from build123d import *

# Parameters (mm, degrees)
SKETCH1_W           = 863.6
SKETCH1_H           = 88.9
BOSS_EXTRUDE1_DEPTH = 38.1
SKETCH3_W           = 88.9
SKETCH3_H           = 38.1
CUT_EXTRUDE1_DEPTH  = 39.1
SKETCH4_W           = 180.975
SKETCH4_H           = 19.05
CUT_EXTRUDE2_DEPTH  = 39.1


with BuildPart() as part:
    # Sketch1 → Boss-Extrude1 (new body)
    with BuildSketch(Plane(origin=(0, 0, 0), x_dir=(1, 0, 0), z_dir=(0, 1, 0))):
        with Locations((431.8, 44.45)):
            Rectangle(SKETCH1_W, SKETCH1_H)
    extrude(amount=BOSS_EXTRUDE1_DEPTH)

    # Sketch3 → Cut-Extrude1 (cut, through all)
    with BuildSketch(Plane(origin=(0, 38.1, 0), x_dir=(1, 0, 0), z_dir=(0, 1, 0))):
        with Locations((44.45, 69.85)):
            Rectangle(SKETCH3_W, SKETCH3_H)
        with Locations((819.15, 69.85)):
            Rectangle(SKETCH3_W, SKETCH3_H)
    extrude(amount=-CUT_EXTRUDE1_DEPTH, mode=Mode.SUBTRACT)

    # Sketch4 → Cut-Extrude2 (cut, through all)
    with BuildSketch(Plane(origin=(0, 38.1, 0), x_dir=(1, 0, 0), z_dir=(0, 1, 0))):
        with Locations((773.1125, 9.525)):
            Rectangle(SKETCH4_W, SKETCH4_H)
    extrude(amount=-CUT_EXTRUDE2_DEPTH, mode=Mode.SUBTRACT)


solid = part.part
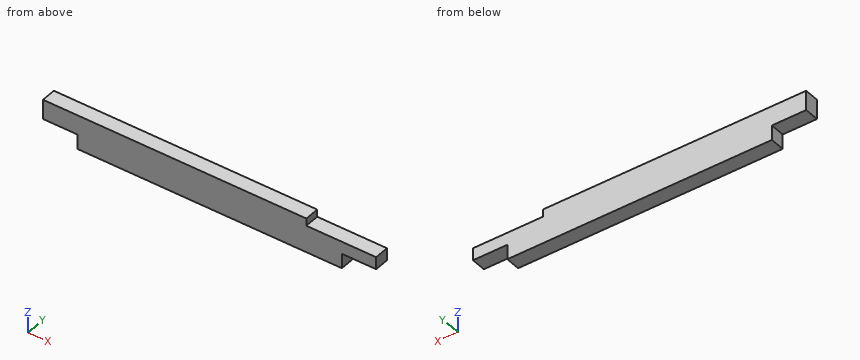
Could you check a few things on this model? Use its own coordinates, in mm. Give positions to 0.01 mm unless a question says otherwise; leave off trailing zeros. Order: outer loops, then holes, each group sorted by start corner. A loop starts at its lowest first (then second) coordinate and runs counter-clockwise, first axis right, second up.
1. Suppose I cut it at B-B (x = 794). List the corners of the cut face in (y, z) for me, plus the area to 3 significant figures.
2. Suppose I cut it at A-A (y = 24). List the corners of the cut face in (x, z) for me (3 decimals), plus the area to 3 significant figures.
3. I need wall thicknesses on L1, parallel to X at y = 2, z = -5 (3 decimals); L2, parallel to X at y = 23.5, z = -78.5; L3, parallel to Z at x = 712, y = 16. Which ranges of each line are inside material? Lowest first, please.
4. Will these pins go through, and if not, where does the flat tip stop? P1, Ø4, axis at x = 756.5, y = 31, coming from the +Z side; P2, Ø6, axis at y = 32, z = -55.5, coming from the -X side; P3, Ø15, axis at y = 10.5, z = -9.5, coming from the +X side (3 decimals).
5. Suppose I cut it at C-C (z = -11). List the corners of the cut face in (x, y) for me (3 decimals), plus the area to 3 significant figures.
Solved:
1. outline: (0, -50.8) - (38.1, -50.8) - (38.1, -19.05) - (0, -19.05) - close
1. area: 1,210 mm2
2. outline: (0, -50.8) - (88.9, -50.8) - (88.9, -88.9) - (774.7, -88.9) - (774.7, -50.8) - (863.6, -50.8) - (863.6, -19.05) - (682.625, -19.05) - (682.625, 0) - (0, 0) - close
2. area: 66,600 mm2
3. L1: x = 0 to 682.625
3. L2: x = 88.9 to 774.7
3. L3: z = -88.9 to -19.05
4. P1: stops at z = -19.05
4. P2: stops at x = 88.9
4. P3: stops at x = 682.625
5. outline: (0, 0) - (682.625, 0) - (682.625, 38.1) - (0, 38.1) - close
5. area: 26,000 mm2
